```python
from build123d import *

# Parameters (mm, degrees)
SKETCH1_W                = 76.2
SKETCH1_H                = 76.2
BOSS_EXTRUDE1_DEPTH      = 101.6
BOSS_EXTRUDE2_DEPTH      = 38.1
BOSS_EXTRUDE2_DEPTH_BACK = 38.1
SKETCH2_R                = 38.1
CUT_EXTRUDE1_DEPTH       = 150.730791756
CUT_EXTRUDE1_DEPTH_BACK  = 150.730791756
SKETCH3_W                = 27.94
SKETCH3_H                = 27.94
SKETCH4_R                = 12.7
BOSS_EXTRUDE3_DEPTH      = 88.9


with BuildPart() as part:
    # Sketch1 → Boss-Extrude1 (new body)
    with BuildSketch(Plane(origin=(0, 0, 0), x_dir=(1, 0, 0), z_dir=(0, 1, 0))):
        Rectangle(SKETCH1_W, SKETCH1_H)
    extrude(amount=BOSS_EXTRUDE1_DEPTH)

    # Sketch2 → Boss-Extrude2 (add, two sides: drawn at the far end of the back side and taken through both)
    with BuildSketch(Plane.XY.offset(-BOSS_EXTRUDE2_DEPTH_BACK)):
        with Locations((0, 101.6)):
            Circle(SKETCH2_R)
    extrude(amount=BOSS_EXTRUDE2_DEPTH + BOSS_EXTRUDE2_DEPTH_BACK)

    # Sketch3 → Cut-Extrude1 (cut, two sides: drawn at the far end of the back side and taken through both)
    with BuildSketch(Plane.XY.offset(-CUT_EXTRUDE1_DEPTH_BACK)):
        with Locations((0, 39.37)):
            Rectangle(SKETCH3_W, SKETCH3_H)
    extrude(amount=CUT_EXTRUDE1_DEPTH + CUT_EXTRUDE1_DEPTH_BACK, mode=Mode.SUBTRACT)

    # Sketch4 → Boss-Extrude3 (add)
    with BuildSketch(Plane.XY):
        with Locations(Location((0, 101.6, 0), (0, 0, 180))):
            Circle(SKETCH4_R)
    extrude(amount=BOSS_EXTRUDE3_DEPTH)


solid = part.part
```
For this review, take the finished solid that the model builds, in its own axes (mm). A direction names the side the tool comes from. Round coordinates to 2 decimals unless told otherwise and drop trailing zeros. Order: outer loops, then holes, each group sorted by start corner. A loop starts at its lowest first (then second) coordinate and runs counter-clockwise, first axis right, second up.
Q1. We need section B-B, the plane z = 17.5. Give the boundary of the cut face in (x, y), plus the area to 3 significant figures.
Findings below:
outline: (-38.1, 0) - (38.1, 0) - (38.1, 101.6) arc R38.1 ccw to (-38.1, 101.6) - close; hole (-13.97, 25.4) - (13.97, 25.4) - (13.97, 53.34) - (-13.97, 53.34) - close
area: 9,240 mm2
Q2. Insertion check: P1, Ø4, axis at x = 30, z = -21.5, coming from the +Y side; P2, Ø22.5, axis at x = -3.5, z = 12.5, coming from the +Y side; P3, Ø2, axis at y = 121, z = 21.5, coming from the +X side; P4, Ø8, axis at y = 21, z = 44, coming from the +X side. Each pin has a flat end and moves straight along its axis. Give the tip position at first contact, or say it passes through.
Findings below:
P1: stops at y = 127.44
P2: stops at y = 139.7
P3: stops at x = 33.36
P4: passes through
Q3. Mouldability with a two-part tool opening along X and no side actions: class faces 1 (the flat face through (13.97, 39, -1)), 2 (the flat face through (-1, 69, 38.1)), 3 (the cylindrical face through (0.84, 139.69, -0.53)) as pulls with the +X half, pulls with the -X half, needs draft (parallel to the pull), parting line crosses it, or undercut.
Findings below:
face 1: undercut
face 2: needs draft
face 3: parting line crosses it
Q4. Wall thickness on line 1 (X direction, y = 37.5, z = 36); line 2 (Y direction, x = 1, z = 69.5); line 3 (Z direction, x = 17, y = 11): over which ranges is each line inside the solid? List them lowest first.
Findings below:
line 1: x = -38.1 to -13.97, 13.97 to 38.1
line 2: y = 88.94 to 114.26
line 3: z = -38.1 to 38.1
Q5. Machinability: for faces 4 (the flat face through (0, 101, 88.9)), 5 (the cylindrical face through (1.653, 89.008, 63.144)), 6 (the flat face through (0, 25.4, -1)), which of the approach directions +Z, -Z, +X, -X, +Y, -Y give a long, thin tool a straight path to every point of the face, cutting with its end or side? Answer none if there is none.
Findings below:
face 4: +Z, +X, -X, +Y, -Y
face 5: +Z
face 6: +Z, -Z
Q6. We need section C-C, the plane y = 92. Give the boundary of the cut face in (x, z), plus the area to 3 significant figures.
Findings below:
outline: (-38.1, -38.1) - (38.1, -38.1) - (38.1, 38.1) - (8.31, 38.1) - (8.31, 88.9) - (-8.31, 88.9) - (-8.31, 38.1) - (-38.1, 38.1) - close
area: 6,650 mm2
Q7. We need section A-A, the plane x = 0. Give the boundary of the cut face in (y, z).
Findings below:
outline: (0, -38.1) - (25.4, -38.1) - (25.4, 38.1) - (0, 38.1) - close; (53.34, -38.1) - (139.7, -38.1) - (139.7, 38.1) - (114.3, 38.1) - (114.3, 88.9) - (88.9, 88.9) - (88.9, 38.1) - (53.34, 38.1) - close
Q8. We need section D-D, the plane z = 78. Give the boundary of the cut face in (x, y), plus the area to 3 significant figures.
Findings below:
outline: circle Ø25.4 at (0, 101.6)
area: 507 mm2
